Work out the finished part from the listing and answer in its coordinate system (mm). A direction names the side the tool comes from. Round coordinates to 2 decimals unless told otherwise and drop trailing zeros. Write each loop counter-clockwise with the first axis right and the second up, starting at its lowest first coordinate (ties: lowest second). Pieces come first, ordered by that corner, then holes. Notation, with made-up numbers: (78, 63.5) - (97, 63.5) arc R23 ccw to (97, 96.5) - close; hole circle Ø11 at (48.25, 26.25). An arc over 180 degrees is marked (long way). Answer as a JSON object with one key per item and string values.
```python
from build123d import *

# Parameters (mm, degrees)
SKETCH_2_W          = 23
SKETCH_2_H          = 12
EXTRUDE_1_DEPTH     = 27
EXTRUDE_START       = -6
SKETCH_3_W          = 32
SKETCH_3_H          = 12
EXTRUDE_2_DEPTH     = 1.2
SKETCH_4_R          = 2.5
EXTRUDE_3_DEPTH     = 4
SKETCH_5_R          = 1
CUT_EXTRUDE_1_DEPTH = 4


with BuildPart() as part:
    # 草图2 → 凸台-拉伸1 (new body)
    with BuildSketch(Plane.XY):
        Rectangle(SKETCH_2_W, SKETCH_2_H)
    extrude(amount=EXTRUDE_1_DEPTH)

    # 草图3 → 凸台-拉伸2 (add)
    with BuildSketch(Plane.XY.offset(27).offset(EXTRUDE_START)):
        Rectangle(SKETCH_3_W, SKETCH_3_H)
    extrude(amount=-EXTRUDE_2_DEPTH)

    # 草图4 → 凸台-拉伸3 (add)
    with BuildSketch(Plane.XY.offset(27)):
        with Locations(Location((-5.5, 0, 0), (0, 0, 180))):
            Circle(SKETCH_4_R)
    extrude(amount=EXTRUDE_3_DEPTH)

    # 草图5 → 切除-拉伸1 (cut)
    with BuildSketch(Plane.XY.offset(21)):
        with Locations((14, 3.25)):
            Circle(SKETCH_5_R)
        with Locations((14, -3.25)):
            Circle(SKETCH_5_R)
        with Locations((-14, -3.25)):
            Circle(SKETCH_5_R)
        with Locations((-14, 3.25)):
            Circle(SKETCH_5_R)
    extrude(amount=-CUT_EXTRUDE_1_DEPTH, mode=Mode.SUBTRACT)


solid = part.part
```
Item 1: Each of these flat-tipped pins is pushed along its axis until it touches: P1, Ø3.5, axis at x = 5, y = 2.5, coming from the +Z side; P2, Ø3, axis at y = 2.5, z = 24.5, coming from the +X side; P3, Ø2.5, axis at x = 14, y = 3.25, coming from the -Z side; P4, Ø3.5, axis at x = -13, y = 1.5, coming from the -Z side. Where does it stop, or does it pass through?
Results found:
{"P1": "z = 27", "P2": "x = 11.5", "P3": "z = 19.8", "P4": "z = 0"}
Item 2: Determine the mould class of faces 6 (the flat face through (0, 6, 14)), 7 (the cylindrical face through (-13.046, -2.95, 20.408)), 8 (the flat face through (14, 0, 19.8)) for opening direction Y: pulls with the +Y half, pulls with the -Y half, needs draft (parallel to the pull), parting line crosses it, or undercut.
Results found:
{"face 6": "pulls with the +Y half", "face 7": "undercut", "face 8": "needs draft"}
Item 3: A cutting plane is placed at C-C (y = 5). Write down the section's boundary in (x, z), and give its area (3 significant figures).
Results found:
{"outline": "(-16, 19.8) - (-11.5, 19.8) - (-11.5, 0) - (11.5, 0) - (11.5, 19.8) - (16, 19.8) - (16, 21) - (11.5, 21) - (11.5, 27) - (-11.5, 27) - (-11.5, 21) - (-16, 21) - close", "area": "632 mm²"}
Item 4: A cutting plane is placed at D-D (x = -5.5). Write down the section's boundary in (y, z), and give its area (3 significant figures).
Results found:
{"outline": "(-6, 0) - (6, 0) - (6, 27) - (2.5, 27) - (2.5, 31) - (-2.5, 31) - (-2.5, 27) - (-6, 27) - close", "area": "344 mm²"}
Item 5: A cutting plane is placed at A-A (y = -3.25). Write down the section's boundary in (x, z), and give its area (3 significant figures).
Results found:
{"outline": "(-16, 19.8) - (-15, 19.8) - (-15, 21) - (-16, 21) - close; (-13, 19.8) - (-11.5, 19.8) - (-11.5, 0) - (11.5, 0) - (11.5, 19.8) - (13, 19.8) - (13, 21) - (11.5, 21) - (11.5, 27) - (-11.5, 27) - (-11.5, 21) - (-13, 21) - close; (15, 19.8) - (16, 19.8) - (16, 21) - (15, 21) - close", "area": "627 mm²"}
Item 6: Consider line 1 along Y through (x, z) = (-14, 20); line 2 along X through (y, z) = (4.75, 15); line 3 along Z through (x, y) = (-9.5, -1.5). Determine where each line is inside the solid, lowest interval first.
Results found:
{"line 1": "-6 to -4.25, -2.25 to 2.25, 4.25 to 6", "line 2": "-11.5 to 11.5", "line 3": "0 to 27"}
Item 7: A cutting plane is placed at B-B (x = -14). Write down the section's boundary in (y, z), and give its area (3 significant figures).
Results found:
{"outline": "(-6, 19.8) - (-4.25, 19.8) - (-4.25, 21) - (-6, 21) - close; (-2.25, 19.8) - (2.25, 19.8) - (2.25, 21) - (-2.25, 21) - close; (4.25, 19.8) - (6, 19.8) - (6, 21) - (4.25, 21) - close", "area": "9.60 mm²"}
Item 8: For faces 1 (the flat face through (-11.5, 0, 10)), 2 (the flat face through (14, 0, 21)), 3 (the cylindrical face through (-7.885, -0.751, 28.972)), 4 (the flat face through (11.5, 0, 10)), 5 (the flat face through (-14, 0, 21)), determine the directions among +Z, -Z, +X, -X, +Y, -Y from which every point of the face is accessible in a straight line to the end or side of a thin tool.
Results found:
{"face 1": "-Z, -X, +Y, -Y", "face 2": "+Z, +X, +Y, -Y", "face 3": "+Z", "face 4": "-Z, +X, +Y, -Y", "face 5": "+Z, -X, +Y, -Y"}
